CAD build for the part. Positions are in the model's coordinates, mm. A direction names the side the tool comes from. Coordinates: 2 decimals unless noted, no trailing zeros. Write each loop counter-clockwise with the first axis right and the second up, starting at its lowest first coordinate (ties: lowest second). Pieces come first, ordered by that corner, then holes. Notation, with made-up numbers: (6.25, 10.5) -> (11.25, 10.5) arc R9 ccw to (11.25, 26.5) -> close; hole circle Ø4 at (-5.5, 81). An arc over 180 degrees is marked (long way). Answer as CSV lines item,"result". Start each with the question number.
```python
from build123d import *

# Parameters (mm, degrees)
BASE_DEPTH        = 1
INT_RIEUR_DEPTH   = 1.8
PASSAGE_VIS_REACH = 25.751
ESQUISSE4_R       = 1.55
ESQUISSE5_W       = 27.6
ESQUISSE5_H       = 42.6
CLEANING_DEPTH    = 1.8


with BuildPart() as part:
    # Esquisse1 → Base (new body)
    with BuildSketch(Plane(origin=(0, 0, 0), x_dir=(1, 0, 0), z_dir=(0, 1, 0))):
        with BuildLine():
            Line((-10.5, 20), (10.5, 20))
            ThreePointArc((10.5, 20), (11.914213562, 19.414213562), (12.5, 18))
            Line((12.5, 18), (12.5, -18))
            ThreePointArc((12.5, -18), (11.914213562, -19.414213562), (10.5, -20))
            Line((10.5, -20), (-10.5, -20))
            ThreePointArc((-10.5, -20), (-11.914213562, -19.414213562), (-12.5, -18))
            Line((-12.5, -18), (-12.5, 18))
            ThreePointArc((-12.5, 18), (-11.914213562, 19.414213562), (-10.5, 20))
        make_face()
    extrude(amount=BASE_DEPTH)

    # Esquisse2 → Intérieur (add)
    with BuildSketch(Plane(origin=(0, 1, 0), x_dir=(1, 0, 0), z_dir=(0, 1, 0))):
        with BuildLine():
            Line((10.5, 18.3), (-10.5, 18.3))
            ThreePointArc((-10.5, 18.3), (-10.712132034, 18.212132034), (-10.8, 18))
            Line((-10.8, 18), (-10.8, -18))
            ThreePointArc((-10.8, -18), (-10.712132034, -18.212132034), (-10.5, -18.3))
            Line((-10.5, -18.3), (10.5, -18.3))
            ThreePointArc((10.5, -18.3), (10.712132034, -18.212132034), (10.8, -18))
            Line((10.8, -18), (10.8, 18))
            ThreePointArc((10.8, 18), (10.712132034, 18.212132034), (10.5, 18.3))
        make_face()
        with BuildLine():
            Line((-6.9, 14.8), (6.9, 14.8))
            ThreePointArc((6.9, 14.8), (7.182842712, 14.682842712), (7.3, 14.4))
            Line((7.3, 14.4), (7.3, -14.4))
            ThreePointArc((7.3, -14.4), (7.182842712, -14.682842712), (6.9, -14.8))
            Line((6.9, -14.8), (-6.9, -14.8))
            ThreePointArc((-6.9, -14.8), (-7.182842712, -14.682842712), (-7.3, -14.4))
            Line((-7.3, -14.4), (-7.3, 14.4))
            ThreePointArc((-7.3, 14.4), (-7.182842712, 14.682842712), (-6.9, 14.8))
        make_face(mode=Mode.SUBTRACT)
    extrude(amount=INT_RIEUR_DEPTH)

    # Esquisse4 → Passage_Vis (cut, up to next)
    with BuildSketch(Plane.XZ, mode=Mode.PRIVATE) as passage_vis_sk1:
        with Locations(Location((-9.5, 17, 0), (0, 0, 270))):
            Circle(ESQUISSE4_R)
    passage_vis_tool1 = extrude(passage_vis_sk1.sketch, amount=-PASSAGE_VIS_REACH, mode=Mode.PRIVATE) & part.part
    # Esquisse4 → Passage_Vis (cut, up to next)
    with BuildSketch(Plane.XZ, mode=Mode.PRIVATE) as passage_vis_sk2:
        with Locations(Location((9.5, 17, 0), (0, 0, 327.004114526))):
            Circle(ESQUISSE4_R)
    passage_vis_tool2 = extrude(passage_vis_sk2.sketch, amount=-PASSAGE_VIS_REACH, mode=Mode.PRIVATE) & part.part
    # Esquisse4 → Passage_Vis (cut, up to next)
    with BuildSketch(Plane.XZ, mode=Mode.PRIVATE) as passage_vis_sk3:
        with Locations(Location((9.5, -17, 0), (0, 0, 270))):
            Circle(ESQUISSE4_R)
    passage_vis_tool3 = extrude(passage_vis_sk3.sketch, amount=-PASSAGE_VIS_REACH, mode=Mode.PRIVATE) & part.part
    # Esquisse4 → Passage_Vis (cut, up to next)
    with BuildSketch(Plane.XZ, mode=Mode.PRIVATE) as passage_vis_sk4:
        with Locations(Location((-9.5, -17, 0), (0, 0, 237.004114526))):
            Circle(ESQUISSE4_R)
    passage_vis_tool4 = extrude(passage_vis_sk4.sketch, amount=-PASSAGE_VIS_REACH, mode=Mode.PRIVATE) & part.part
    add(passage_vis_tool1.solids().sort_by_distance((-9.5, 0, 17))[0], mode=Mode.SUBTRACT)
    add(passage_vis_tool2.solids().sort_by_distance((9.5, 0, 17))[0], mode=Mode.SUBTRACT)
    add(passage_vis_tool3.solids().sort_by_distance((9.5, 0, -17))[0], mode=Mode.SUBTRACT)
    add(passage_vis_tool4.solids().sort_by_distance((-9.5, 0, -17))[0], mode=Mode.SUBTRACT)

    # Esquisse5 → Cleaning (cut)
    with BuildSketch(Plane(origin=(0, 2.8, 0), x_dir=(1, 0, 0), z_dir=(0, 1, 0))):
        Rectangle(ESQUISSE5_W, ESQUISSE5_H)
        with BuildLine():
            Line((-9.2, 18.3), (9.2, 18.3))
            ThreePointArc((9.2, 18.3), (10.33137085, 17.83137085), (10.8, 16.7))
            Line((10.8, 16.7), (10.8, -16.7))
            ThreePointArc((10.8, -16.7), (10.33137085, -17.83137085), (9.2, -18.3))
            Line((9.2, -18.3), (-9.2, -18.3))
            ThreePointArc((-9.2, -18.3), (-10.33137085, -17.83137085), (-10.8, -16.7))
            Line((-10.8, -16.7), (-10.8, 16.7))
            ThreePointArc((-10.8, 16.7), (-10.33137085, 17.83137085), (-9.2, 18.3))
        make_face(mode=Mode.SUBTRACT)
    extrude(amount=-CLEANING_DEPTH, mode=Mode.SUBTRACT)


solid = part.part
```
1. Cut at C-C (y = 0.5). Give the cut face in (x, z).
2. Tool access for faces 4 (the face through (0, 2, -18.3)), 5 (the face through (-10, 2.8, 0)), 6 (the face through (0, 2, 18.3)), 7 (the face through (0, 1, 0)): list every direction of +Z, -Z, +X, -X, +Y, -Y with a clear straight run to the whole face (end or side of a thin tool).
3. Cut at A-A (z = 17). Give the cut face in (x, y).
4. Mould opens along Z. For faces 1 (the face through (12.5, 0.5, -0.3)), 2 (the face through (-11.9, 0.49, 19.43)), 3 (the face through (-8.19, 1.07, 16.17)) say: pulls with the +Z half, pulls with the -Z half, needs draft (parallel to the pull), parting line crosses it, or undercut.
5. Cut at D-D (x = 4.5). Give the cut face in (y, z).
6. Flat gauge pins, fed straight in: P1, Ø0.5, axis at y = 1.5, z = 3, coming from the +X side; P2, Ø0.9, axis at y = 2, z = 6, coming from the -X side; P3, Ø1.4, axis at x = -0.5, y = 2, coming from the +Z side. Where does each tip first touch, or does it go through?
7. Cut at B-B (x = -9.5). Give the cut face in (y, z), then the cut area to 3 significant figures.
8. Wall check: line 1 (Z direction, x = 9.5, y = 0.8); line 2 (X direction, y = 2, z = 0); line 3 (Z direction, x = -0.5, y = 1.8). Give the ranges that are in metal, low to high.
Geometry check:
1,outline,"(-12.5, -18) arc R2 ccw to (-10.5, -20) -> (10.5, -20) arc R2 ccw to (12.5, -18) -> (12.5, 18) arc R2 ccw to (10.5, 20) -> (-10.5, 20) arc R2 ccw to (-12.5, 18) -> close; hole circle Ø3.1 at (-9.5, -17); hole circle Ø3.1 at (-9.5, 17); hole circle Ø3.1 at (9.5, -17); hole circle Ø3.1 at (9.5, 17)"
2,face 4,"-Z, +X, -X, +Y"
2,face 5,"+Z, -Z, +X, -X, +Y"
2,face 6,"+Z, +X, -X, +Y"
2,face 7,"+Y"
3,outline,"(-12.5, 0) -> (-11.05, 0) -> (-11.05, 1) -> (-12.5, 1) -> close; (-7.95, 0) -> (7.95, 0) -> (7.95, 2.8) -> (-7.95, 2.8) -> close; (11.05, 0) -> (12.5, 0) -> (12.5, 1) -> (11.05, 1) -> close"
4,face 1,"needs draft"
4,face 2,"pulls with the +Z half"
4,face 3,"undercut"
5,outline,"(0, -20) -> (1, -20) -> (1, -18.3) -> (2.8, -18.3) -> (2.8, -14.8) -> (1, -14.8) -> (1, 14.8) -> (2.8, 14.8) -> (2.8, 18.3) -> (1, 18.3) -> (1, 20) -> (0, 20) -> close"
6,P1,"x = 10.8"
6,P2,"x = -10.8"
6,P3,"z = 18.3"
7,outline,"(0, -20) -> (1, -20) -> (1, -18.55) -> (0, -18.55) -> close; (0, -15.45) -> (2.8, -15.45) -> (2.8, 15.45) -> (0, 15.45) -> close; (0, 18.55) -> (1, 18.55) -> (1, 20) -> (0, 20) -> close"
7,area,"89.4 mm²"
8,line 1,"-20 to -18.55, -15.45 to 15.45, 18.55 to 20"
8,line 2,"-10.8 to -7.3, 7.3 to 10.8"
8,line 3,"-18.3 to -14.8, 14.8 to 18.3"
